Design review of the part shown in the three views and the two pictorial views. Dimensions are in mm from the part's minimum x, y and z. A direction names the side the tool comes from. Give positions to 0.01 mm unless a question says otherwise; leave off trailing zeros. Order: outer loops, then holes, each group sorted by start corner. A loop starts at its lowest first (then second) coordinate and runs counter-clockwise, first axis right, second up. Notation, with made-up numbers: (-19, 16.5) - (36, 16.5) arc R38 cw to (36, 55.5) - close; hole circle Ø1 at (86, 68). An arc over 180 degrees is marked (long way). Put each result on its own line as item: value.
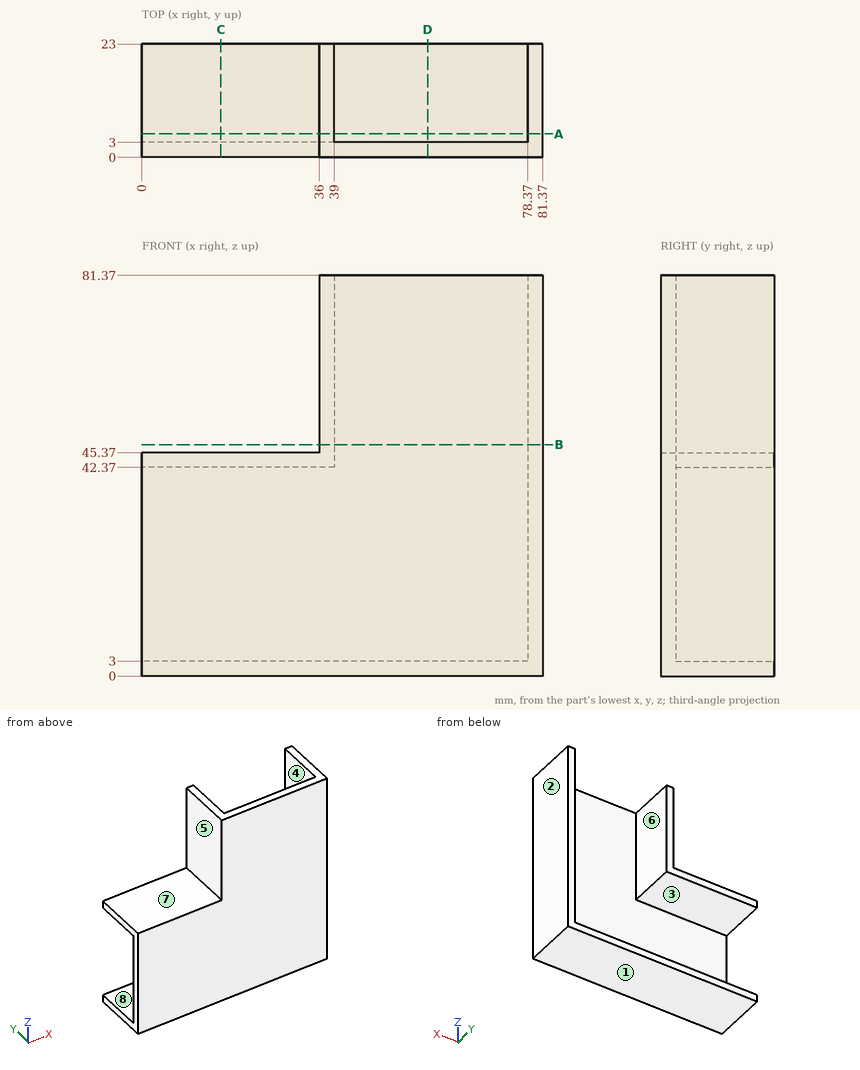
(1) Take a section at A-A, the plane y = 4.75. Write out the cut boundary in (x, z), then the cut area to 3 significant figures.
The answers:
outline: (0, 0) - (81.37, 0) - (81.37, 81.37) - (78.37, 81.37) - (78.37, 3) - (0, 3) - close; (0, 42.37) - (39, 42.37) - (39, 81.37) - (36, 81.37) - (36, 45.37) - (0, 45.37) - close
area: 704 mm^2
(2) Wall thickness on L1, parallel to Z at x = 25.5, y = 17; L2, parallel to X at y = 21.25, z = 74.5; L3, parallel to Y at x = 74.5, z = 42.5: over which ranges is each line inside the solid? List them lowest first.
The answers:
L1: 0 to 3, 42.37 to 45.37
L2: 36 to 39, 78.37 to 81.37
L3: 0 to 3
(3) For the marked faces 1, 2, 3, 4 and 5, list the 3-axis set-ups (+Z, -Z, +X, -X, +Y, -Y) from which the entire face can be reached by the end or side of a thin tool; tool diameter is ignored.
The answers:
face 1: -Z, +X, -X, +Y, -Y
face 2: +Z, -Z, +X, +Y, -Y
face 3: -X, +Y
face 4: +Z, +Y
face 5: +Z, -X, +Y, -Y
(4) Clearance check with flat-ended pins moving along their axes: pin 1 Ø10 at (x, y) = (51, 15.5) entering from +Z; pin 2 Ø5 at (x, z) = (48, 14.5) entering from +Y; pin 3 Ø8 at (y, z) = (20, 22.5) entering from -X. State where each tip first meets the part, or that it passes through.
The answers:
pin 1: z = 3
pin 2: y = 3
pin 3: x = 78.37
(5) Take a section at D-D, the plane x = 58. Write out the cut boundary in (y, z).
The answers:
outline: (0, 0) - (23, 0) - (23, 3) - (3, 3) - (3, 81.37) - (0, 81.37) - close
(6) Take a section at B-B, the plane z = 47. Write out the cut boundary in (x, y), then the cut area to 3 significant figures.
The answers:
outline: (36, 0) - (81.37, 0) - (81.37, 23) - (78.37, 23) - (78.37, 3) - (39, 3) - (39, 23) - (36, 23) - close
area: 256 mm^2
(7) The part is to be moulded in two halves that separate along Z. For the marked faces 6, 7 and 8, say which applies: pulls with the +Z half, pulls with the -Z half, needs draft (parallel to the pull), parting line crosses it, or undercut.
The answers:
face 6: needs draft
face 7: pulls with the +Z half
face 8: undercut
(8) Take a section at C-C, the plane x = 16. Write out the cut boundary in (y, z).
The answers:
outline: (0, 0) - (23, 0) - (23, 3) - (3, 3) - (3, 42.37) - (23, 42.37) - (23, 45.37) - (0, 45.37) - close
